from build123d import *

# Parameters (mm, degrees)
F0_W     = 300
F0_H     = 135
F1_DEPTH = 410
F2_W     = 68.75
F2_H     = 45.625
F3_DEPTH = 125


with BuildPart() as f1:
    # F0 (on Top) → F1 (new body)
    with BuildSketch(Plane.XY):
        with Locations((150, 67.5)):
            Rectangle(F0_W, F0_H)
    extrude(amount=F1_DEPTH)

    # F2 (on face) → F3 (cut)
    with BuildSketch(Plane.XZ):
        with Locations((260.625, 230.3125)):
            Rectangle(F2_W, F2_H)
        with Locations((260.625, 280.9375)):
            Rectangle(F2_W, F2_H)
        with Locations((260.625, 331.5625)):
            Rectangle(F2_W, F2_H)
        with Locations((260.625, 382.1875)):
            Rectangle(F2_W, F2_H)
        with Locations((186.875, 382.1875)):
            Rectangle(F2_W, F2_H)
        with Locations((113.125, 382.1875)):
            Rectangle(F2_W, F2_H)
        with Locations((260.625, 179.6875)):
            Rectangle(F2_W, F2_H)
        with Locations((260.625, 129.0625)):
            Rectangle(F2_W, F2_H)
        with Locations((260.625, 78.4375)):
            Rectangle(F2_W, F2_H)
        with Locations((260.625, 27.8125)):
            Rectangle(F2_W, F2_H)
        with Locations((186.875, 27.8125)):
            Rectangle(F2_W, F2_H)
        with Locations((113.125, 27.8125)):
            Rectangle(F2_W, F2_H)
        with Locations((39.375, 27.8125)):
            Rectangle(F2_W, F2_H)
        with Locations((39.375, 78.4375)):
            Rectangle(F2_W, F2_H)
        with Locations((39.375, 129.0625)):
            Rectangle(F2_W, F2_H)
        with Locations((39.375, 179.6875)):
            Rectangle(F2_W, F2_H)
        with Locations((39.375, 230.3125)):
            Rectangle(F2_W, F2_H)
        with Locations((39.375, 280.9375)):
            Rectangle(F2_W, F2_H)
        with Locations((39.375, 331.5625)):
            Rectangle(F2_W, F2_H)
        with Locations((39.375, 382.1875)):
            Rectangle(F2_W, F2_H)
        with Locations((113.125, 331.5625)):
            Rectangle(F2_W, F2_H)
        with Locations((113.125, 280.9375)):
            Rectangle(F2_W, F2_H)
        with Locations((113.125, 230.3125)):
            Rectangle(F2_W, F2_H)
        with Locations((186.875, 331.5625)):
            Rectangle(F2_W, F2_H)
        with Locations((186.875, 280.9375)):
            Rectangle(F2_W, F2_H)
        with Locations((186.875, 230.3125)):
            Rectangle(F2_W, F2_H)
        with Locations((186.875, 78.4375)):
            Rectangle(F2_W, F2_H)
        with Locations((113.125, 78.4375)):
            Rectangle(F2_W, F2_H)
        with Locations((113.125, 129.0625)):
            Rectangle(F2_W, F2_H)
        with Locations((186.875, 129.0625)):
            Rectangle(F2_W, F2_H)
        with Locations((113.125, 179.6875)):
            Rectangle(F2_W, F2_H)
        with Locations((186.875, 179.6875)):
            Rectangle(F2_W, F2_H)
    extrude(amount=-F3_DEPTH, mode=Mode.SUBTRACT)


solid = f1.part
Design review of the part built by this model. Coordinates are the model's own, in mm. Give positions to 0.01 mm unless a question says otherwise; leave off trailing zeros. Loops run counter-clockwise (first coordinate to the right, second up) from the corner with the lowest first, then second, coordinate; pieces in that order, holes last. Notation, with made-up numbers: (74.25, 88) - (103.25, 88) arc R28 cw to (103.25, 124) - close; hole circle Ø5 at (8, 9). An arc over 180 degrees is marked (long way). Use CSV: the item, a comma, the result in double quotes. Start each with the question number.
1. Add section A-A (z = 114). State the section outline as (x, y) points.
2. Add section B-B (y = 14.5). Count the separate pieces of the cut face and the enclosed holes in it, plus the area to 3 significant figures.
3. Wall thickness on L1, parallel to X at y = 59.5, z = 390; L2, parallel to Y at x = 258, z = 86.5: over which ranges is each line inside the solid? List them lowest first.
4. Insertion check: P1, Ø13.5, axis at x = 34.5, z = 290.5, coming from the -Y side; P2, Ø6, axis at x = 157, y = 75.5, coming from the -Z side. Each pin has a flat end and moves straight along its axis. Give the tip position at first contact, or say it passes through.
Results found:
1,outline,"(0, 0) - (5, 0) - (5, 125) - (73.75, 125) - (73.75, 0) - (78.75, 0) - (78.75, 125) - (147.5, 125) - (147.5, 0) - (152.5, 0) - (152.5, 125) - (221.25, 125) - (221.25, 0) - (226.25, 0) - (226.25, 125) - (295, 125) - (295, 0) - (300, 0) - (300, 135) - (0, 135) - close"
2,separate pieces,"1"
2,enclosed holes,"32"
2,area,"22,600 mm²"
3,L1,"x = 0 to 5, 73.75 to 78.75, 147.5 to 152.5, 221.25 to 226.25, 295 to 300"
3,L2,"y = 125 to 135"
4,P1,"stops at y = 125"
4,P2,"stops at z = 0"
